Source: CAD feature listing. Evaluate the final solid. Frame: model axes, mm. Coordinates: 2 decimals unless noted, no trailing zeros. Order: outer loops, then holes, each group sorted by start corner. A loop starts at its lowest first (then second) coordinate and runs counter-clockwise, first axis right, second up. Notation, with made-up numbers: (-7, 86.5) - (23, 86.5) arc R22 ccw to (23, 121.5) - close; hole circle Ø7 at (23, 16.25). An arc over 180 degrees is marked (long way). One line per question, with ' | ' between items.
from build123d import *

# Parameters (mm, degrees)
SKETCH1_W                = 2.54
SKETCH1_H                = 2.54
BOSS_EXTRUDE1_DEPTH      = 1.27
BOSS_EXTRUDE1_DEPTH_BACK = 1.27
SKETCH2_W                = 0.64
SKETCH2_H                = 0.64
BOSS_EXTRUDE2_DEPTH      = 7
BOSS_EXTRUDE2_DEPTH_BACK = 7
CHAMFER1_SIZE            = 0.5
CHAMFER1_SIZE2           = 0.08816349
CHAMFER1_PART_2_SIZE     = 0.5
CHAMFER1_PART_2_SIZE2    = 0.08816349
CHAMFER1_PART_3_SIZE     = 0.5
CHAMFER1_PART_3_SIZE2    = 0.08816349
CHAMFER1_PART_4_SIZE     = 0.5
CHAMFER1_PART_4_SIZE2    = 0.08816349
CHAMFER1_PART_5_SIZE     = 0.5
CHAMFER1_PART_5_SIZE2    = 0.08816349
CHAMFER1_PART_6_SIZE     = 0.5
CHAMFER1_PART_6_SIZE2    = 0.08816349
CHAMFER1_PART_7_SIZE     = 0.5
CHAMFER1_PART_7_SIZE2    = 0.08816349
CHAMFER1_PART_8_SIZE     = 0.5
CHAMFER1_PART_8_SIZE2    = 0.08816349
CHAMFER2_SIZE            = 0.5


with BuildPart() as part:
    # Sketch1 → Boss-Extrude1 (new body, two sides)
    with BuildSketch(Plane(origin=(0, 0, 0), x_dir=(1, 0, 0), z_dir=(0, 1, 0))) as boss_extrude1_sk:
        Rectangle(SKETCH1_W, SKETCH1_H)
    extrude(amount=BOSS_EXTRUDE1_DEPTH)
    extrude(boss_extrude1_sk.sketch, amount=-BOSS_EXTRUDE1_DEPTH_BACK)

    # Sketch2 → Boss-Extrude2 (add, two sides)
    with BuildSketch(Plane(origin=(0, 0, 0), x_dir=(1, 0, 0), z_dir=(0, 1, 0))) as boss_extrude2_sk:
        Rectangle(SKETCH2_W, SKETCH2_H)
    extrude(amount=BOSS_EXTRUDE2_DEPTH)
    extrude(boss_extrude2_sk.sketch, amount=-BOSS_EXTRUDE2_DEPTH_BACK)

    # Chamfer1
    chamfer1_edges = [part.edges().sort_by_distance(p)[0] for p in [
        (-0.32, -7, 0),
    ]]
    chamfer1_side = [part.faces().sort_by_distance(p)[0] for p in [
        (-0.32, -4.135, 0),
    ]]
    chamfer(chamfer1_edges, length=CHAMFER1_SIZE, length2=CHAMFER1_SIZE2, reference=chamfer1_side[0])

    # Chamfer1 part 2
    chamfer1_part_2_edges = [part.edges().sort_by_distance(p)[0] for p in [
        (0, -7, -0.32),
    ]]
    chamfer1_part_2_side = [part.faces().sort_by_distance(p)[0] for p in [
        (0, -4.135, -0.32),
    ]]
    chamfer(chamfer1_part_2_edges, length=CHAMFER1_PART_2_SIZE, length2=CHAMFER1_PART_2_SIZE2, reference=chamfer1_part_2_side[0])

    # Chamfer1 part 3
    chamfer1_part_3_edges = [part.edges().sort_by_distance(p)[0] for p in [
        (0.32, -7, 0),
    ]]
    chamfer1_part_3_side = [part.faces().sort_by_distance(p)[0] for p in [
        (0.32, -4.135, 0),
    ]]
    chamfer(chamfer1_part_3_edges, length=CHAMFER1_PART_3_SIZE, length2=CHAMFER1_PART_3_SIZE2, reference=chamfer1_part_3_side[0])

    # Chamfer1 part 4
    chamfer1_part_4_edges = [part.edges().sort_by_distance(p)[0] for p in [
        (0, -7, 0.32),
    ]]
    chamfer1_part_4_side = [part.faces().sort_by_distance(p)[0] for p in [
        (0, -4.135, 0.32),
    ]]
    chamfer(chamfer1_part_4_edges, length=CHAMFER1_PART_4_SIZE, length2=CHAMFER1_PART_4_SIZE2, reference=chamfer1_part_4_side[0])

    # Chamfer1 part 5
    chamfer1_part_5_edges = [part.edges().sort_by_distance(p)[0] for p in [
        (-0.32, 7, 0),
    ]]
    chamfer1_part_5_side = [part.faces().sort_by_distance(p)[0] for p in [
        (-0.32, 4.135, 0),
    ]]
    chamfer(chamfer1_part_5_edges, length=CHAMFER1_PART_5_SIZE, length2=CHAMFER1_PART_5_SIZE2, reference=chamfer1_part_5_side[0])

    # Chamfer1 part 6
    chamfer1_part_6_edges = [part.edges().sort_by_distance(p)[0] for p in [
        (0, 7, 0.32),
    ]]
    chamfer1_part_6_side = [part.faces().sort_by_distance(p)[0] for p in [
        (0, 4.135, 0.32),
    ]]
    chamfer(chamfer1_part_6_edges, length=CHAMFER1_PART_6_SIZE, length2=CHAMFER1_PART_6_SIZE2, reference=chamfer1_part_6_side[0])

    # Chamfer1 part 7
    chamfer1_part_7_edges = [part.edges().sort_by_distance(p)[0] for p in [
        (0.32, 7, 0),
    ]]
    chamfer1_part_7_side = [part.faces().sort_by_distance(p)[0] for p in [
        (0.32, 4.135, 0),
    ]]
    chamfer(chamfer1_part_7_edges, length=CHAMFER1_PART_7_SIZE, length2=CHAMFER1_PART_7_SIZE2, reference=chamfer1_part_7_side[0])

    # Chamfer1 part 8
    chamfer1_part_8_edges = [part.edges().sort_by_distance(p)[0] for p in [
        (0, 7, -0.32),
    ]]
    chamfer1_part_8_side = [part.faces().sort_by_distance(p)[0] for p in [
        (0, 4.135, -0.32),
    ]]
    chamfer(chamfer1_part_8_edges, length=CHAMFER1_PART_8_SIZE, length2=CHAMFER1_PART_8_SIZE2, reference=chamfer1_part_8_side[0])

    # Chamfer2
    chamfer2_edges = [part.edges().sort_by_distance(p)[0] for p in [
        (-1.27, 0, -1.27),
        (1.27, 0, -1.27),
        (1.27, 0, 1.27),
        (-1.27, 0, 1.27),
    ]]
    chamfer(chamfer2_edges, length=CHAMFER2_SIZE)


solid = part.part
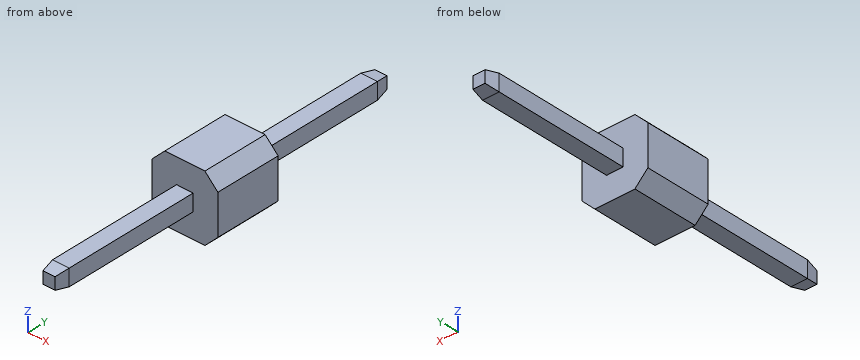
(1) Pin query (flat end, axial travel): P1, Ø0.7, axis at x = 0, y = -3, coming from the +Z side; P2, Ø1.5, axis at x = 0.5, y = 3, coming from the -Z side; P3, Ø0.5, axis at y = 3, z = 0, coming from the +X side. Return the tip coordinate at first contact, or that it passes through.
Taken from the geometry:
P1: stops at z = 0.32 | P2: stops at z = -0.32 | P3: stops at x = 0.32
(2) Material intervals for L1, parallel to X at y = 3.25, z = 0.05; L2, parallel to Y at x = -0.85, z = 0.3, sorted ascending. Write a range as from..to.
Taken from the geometry:
L1: x = -0.32..0.32 | L2: y = -1.27..1.27
(3) Cut plane A-A (x = 0.1). Return the cut outline in (y, z), and give its area (3 significant figures).
Taken from the geometry:
outline: (-7, -0.23) - (-6.5, -0.32) - (-1.27, -0.32) - (-1.27, -1.27) - (1.27, -1.27) - (1.27, -0.32) - (6.5, -0.32) - (7, -0.23) - (7, 0.23) - (6.5, 0.32) - (1.27, 0.32) - (1.27, 1.27) - (-1.27, 1.27) - (-1.27, 0.32) - (-6.5, 0.32) - (-7, 0.23) - close | area: 13.7 mm²
(4) Cut plane B-B (y = 1). Return the cut outline in (x, z).
Taken from the geometry:
outline: (-1.27, -0.77) - (-0.77, -1.27) - (0.77, -1.27) - (1.27, -0.77) - (1.27, 0.77) - (0.77, 1.27) - (-0.77, 1.27) - (-1.27, 0.77) - close
(5) Cut plane C-C (z = -0.1). Return the cut outline in (x, y), and give its area (3 significant figures).
Taken from the geometry:
outline: (-1.27, -1.27) - (-0.32, -1.27) - (-0.32, -6.5) - (-0.23, -7) - (0.23, -7) - (0.32, -6.5) - (0.32, -1.27) - (1.27, -1.27) - (1.27, 1.27) - (0.32, 1.27) - (0.32, 6.5) - (0.23, 7) - (-0.23, 7) - (-0.32, 6.5) - (-0.32, 1.27) - (-1.27, 1.27) - close | area: 13.7 mm²
(6) Cut plane D-D (y = 6.25). Return the cut outline in (x, z), and give its area (3 significant figures).
Taken from the geometry:
outline: (-0.32, -0.32) - (0.32, -0.32) - (0.32, 0.32) - (-0.32, 0.32) - close | area: 0.410 mm²
